```python
from build123d import *

# Parameters (mm, degrees)
SKETCH1_W                 = 47.35
SKETCH1_H                 = 43.25
BOSS_EXTRUDE2_DEPTH       = 2
EDGE_FLANGE1_START        = -2
EDGE_FLANGE1_OUTLINE_W    = 1
EDGE_FLANGE1_OUTLINE_H    = 2
EDGE_FLANGE1_DEPTH        = 2
EDGE_FLANGE1_START_2      = -1
EDGE_FLANGE1_2_DEPTH      = 3.69178
EDGE_FLANGE1_3_OUTLINE_W  = 2
EDGE_FLANGE1_3_OUTLINE_H  = 26.65
EDGE_FLANGE1_3_DEPTH      = 12
EDGE_FLANGE1_START_3      = 8.3
EDGE_FLANGE1_4_DEPTH      = 26.65
EDGE_FLANGE1_5_DEPTH      = 26.65
EDGE_FLANGE1_START_4      = 47.35
EDGE_FLANGE1_6_OUTLINE_R  = 1.6
EDGE_FLANGE1_6_DEPTH      = 2
REDONDEO1_R               = 2
TALADRO_ROSCADO_M31_D     = 2.5
TALADRO_ROSCADO_M31_DEPTH = 8.5
TALADRO_ROSCADO_M31_TIP   = 0.751075774
CROQUIS4_W                = 37.35
CROQUIS4_H                = 34.25
CORTAR_EXTRUIR1_DEPTH     = 67.377594111
CROQUIS14_W               = 2
CROQUIS14_H               = 7.3
SALIENTE_EXTRUIR1_DEPTH   = 1
FILLET1_R                 = 2
REDONDEO2_R               = 5
REDONDEO3_R               = 1


with BuildPart() as part:
    # Sketch1 → Boss-Extrude2 (new body)
    with BuildSketch(Plane.XY):
        with Locations((23.675, 21.625)):
            Rectangle(SKETCH1_W, SKETCH1_H)
    extrude(amount=BOSS_EXTRUDE2_DEPTH)

    # Edge-Flange1: read off the stored shape, not the designer's step
    # Edge-Flange1 outline → Edge-Flange1 (cut)
    with BuildSketch(Plane(origin=(47.35, 0, 2), x_dir=(0, 1, 0), z_dir=(1, 0, 0)).offset(EDGE_FLANGE1_START)):
        with Locations((35.45, -1)):
            Rectangle(EDGE_FLANGE1_OUTLINE_W, EDGE_FLANGE1_OUTLINE_H)
        with Locations((7.8, -1)):
            Rectangle(EDGE_FLANGE1_OUTLINE_W, EDGE_FLANGE1_OUTLINE_H)
    extrude(amount=EDGE_FLANGE1_DEPTH, mode=Mode.SUBTRACT)

    # Edge-Flange1 2 outline → Edge-Flange1 2 (cut)
    with BuildSketch(Plane.XY.offset(EDGE_FLANGE1_START_2)):
        with BuildLine():
            ThreePointArc((45.35, 35.95), (44.85, 35.45), (45.35, 34.95))
            Line((45.35, 34.95), (45.35, 35.95))
        make_face()
        with BuildLine():
            ThreePointArc((45.35, 8.3), (44.85, 7.8), (45.35, 7.3))
            Line((45.35, 7.3), (45.35, 8.3))
        make_face()
    extrude(amount=EDGE_FLANGE1_2_DEPTH, mode=Mode.SUBTRACT)

    # Edge-Flange1 3 outline → Edge-Flange1 3 (add)
    with BuildSketch(Plane.XY):
        with Locations((48.35, 21.625)):
            Rectangle(EDGE_FLANGE1_3_OUTLINE_W, EDGE_FLANGE1_3_OUTLINE_H)
    extrude(amount=EDGE_FLANGE1_3_DEPTH)

    # Edge-Flange1 4 outline → Edge-Flange1 4 (add)
    with BuildSketch(Plane(origin=(0, 0, 0), x_dir=(1, 0, 0), z_dir=(0, 1, 0)).offset(EDGE_FLANGE1_START_3)):
        with BuildLine():
            ThreePointArc((46.35, -2), (47.057106781, -2.292893219), (47.35, -3))
            Line((47.35, -3), (47.35, -2))
            Line((47.35, -2), (46.35, -2))
        make_face()
    extrude(amount=EDGE_FLANGE1_4_DEPTH)

    # Edge-Flange1 5 outline → Edge-Flange1 5 (cut)
    with BuildSketch(Plane(origin=(0, 0, 0), x_dir=(1, 0, 0), z_dir=(0, 1, 0)).offset(EDGE_FLANGE1_START_3)):
        with BuildLine():
            ThreePointArc((46.35, 0), (48.471320344, -0.878679656), (49.35, -3))
            Line((49.35, -3), (49.35, 0))
            Line((49.35, 0), (46.35, 0))
        make_face()
    extrude(amount=EDGE_FLANGE1_5_DEPTH, mode=Mode.SUBTRACT)

    # Edge-Flange1 6 outline → Edge-Flange1 6 (cut)
    with BuildSketch(Plane.YZ.offset(EDGE_FLANGE1_START_4)):
        with Locations((12.3, 8.5)):
            Circle(EDGE_FLANGE1_6_OUTLINE_R)
        with Locations((30.95, 8.5)):
            Circle(EDGE_FLANGE1_6_OUTLINE_R)
    extrude(amount=EDGE_FLANGE1_6_DEPTH, mode=Mode.SUBTRACT)

    # Redondeo1
    redondeo1_edges = [part.edges().sort_by_distance(p)[0] for p in [
        (48.35, 8.3, 12),
        (48.35, 34.95, 12),
    ]]
    fillet(redondeo1_edges, radius=REDONDEO1_R)

    # Taladro roscado M31
    with Locations(Plane(origin=(0, 0, 0), x_dir=(-1, 0, 0), z_dir=(0, 0, -1))):
        with Locations((-44.65, 39.45), (-4, 3.8), (-44.65, 3.8)):
            Hole(TALADRO_ROSCADO_M31_D / 2, depth=TALADRO_ROSCADO_M31_DEPTH)
            with Locations((0, 0, -(TALADRO_ROSCADO_M31_DEPTH + TALADRO_ROSCADO_M31_TIP / 2))):  # 118° drill point
                Cone(0, TALADRO_ROSCADO_M31_D / 2, TALADRO_ROSCADO_M31_TIP, mode=Mode.SUBTRACT)

    # Croquis4 → Cortar-Extruir1 (cut, through all)
    with BuildSketch(Plane.XY.offset(2)):
        with Locations((18.675, 26.125)):
            Rectangle(CROQUIS4_W, CROQUIS4_H)
    extrude(amount=-CORTAR_EXTRUIR1_DEPTH, mode=Mode.SUBTRACT)

    # Croquis14 → Saliente-Extruir1 (add)
    with BuildSketch(Plane(origin=(47.35, 0, 0), x_dir=(0, 0, -1), z_dir=(1, 0, 0))):
        with Locations((-1, 3.65)):
            Rectangle(CROQUIS14_W, CROQUIS14_H)
        with Locations((-1, 39.6)):
            Rectangle(CROQUIS14_W, CROQUIS14_H)
    extrude(amount=SALIENTE_EXTRUIR1_DEPTH)

    # Fillet1
    fillet1_edges = [part.edges().sort_by_distance(p)[0] for p in [
        (0, 9, 1),
        (37.35, 43.25, 1),
        (48.35, 0, 1),
        (48.35, 43.25, 1),
        (0, 0, 1),
    ]]
    fillet(fillet1_edges, radius=FILLET1_R)

    # Redondeo2
    redondeo2_edges = [part.edges().sort_by_distance(p)[0] for p in [
        (37.35, 9, 1),
    ]]
    fillet(redondeo2_edges, radius=REDONDEO2_R)

    # Redondeo3
    redondeo3_edges = [part.edges().sort_by_distance(p)[0] for p in [
        (48.35, 7.3, 1),
        (48.35, 35.95, 1),
    ]]
    fillet(redondeo3_edges, radius=REDONDEO3_R)


solid = part.part
```
The model under review builds one solid part; all positions refer to its coordinate system, in mm. A direction names the side the tool comes from. Give positions to 0.01 mm unless a question says otherwise; leave off trailing zeros. Write each loop counter-clockwise with the first axis right and the second up, starting at its lowest first coordinate (ties: lowest second). Pieces come first, ordered by that corner, then holes. Notation, with made-up numbers: (78.5, 77.5) - (114.5, 77.5) arc R20 ccw to (114.5, 90.5) - close; hole circle Ø11 at (6.5, 86.25). An arc over 180 degrees is marked (long way). Answer in a Markdown table with one row per item. Add a question column.
1. We need section B-B on y = 39.45. Write out the cut boundary in (x, z), then the cut area to 3 significant figures.
2. We need section A-A on x = 4. Write out the cut boundary in (y, z), then the cut area to 3 significant figures.
3. We need section D-D on z = 4. Write out the cut boundary in (x, y).
4. Draft analysis for pull direction X (two halves, no side actions). For faces 5 (the flat face through (29, 7, 0)), 6 (the flat face through (48.35, 4, 1)), 7 (the cylindrical face through (5.19, 4.18, 1.01)), state which applies: +X half, -X half, draft (parallel to the pull), parting line (faces both ways), or undercut.
5. We need section C-C on y = 25.5. Write out the cut boundary in (x, z), then the cut area to 3 significant figures.
6. Wall thickness on line 1 along Y through (x, z) = (44.65, 0.65); line 2 along Z through (x, y) = (16, 7); line 3 along Z through (x, y) = (48.7, 12.3): over which ranges is each line inside the solid? List them lowest first. Write a range as [from, to].
7. Tool access review of faces 1 (the flat face through (46, 35.95, 1)), 2 (the flat face through (37.35, 27, 1)), 3 (the cylindrical face through (48.45, 21.44, 0.86)), 4 (the cylindrical face through (47.75, 0.57, 0.99)): name each direction out of +Z, -Z, +X, -X, +Y, -Y from which nothing blocks a thin tool from reaching the whole face with its end or side.
8. Insertion check: P1, Ø2, axis at x = 47.5, z = 6.5, coming from the +Y side; P2, Ø2, axis at y = 4.5, z = 1, coming from the +X side; P3, Ø6, axis at y = 32.5, z = 10, coming from the -X side; P4, Ø3, axis at y = 37.5, z = 10.5, coming from the +X side. Each pin has a flat end and moves straight along its axis. Give the tip position at first contact, or say it passes through.
Ans:
| question | item | result |
|---|---|---|
| 1 | outline | (37.35, 0) - (43.4, 0) - (43.4, 2) - (37.35, 2) - close; (45.9, 0) - (48.35, 0) - (48.35, 2) - (45.9, 2) - close |
| 1 | area | 17.0 mm^2 |
| 2 | outline | (0, 0) - (2.55, 0) - (2.55, 2) - (0, 2) - close; (5.05, 0) - (9, 0) - (9, 2) - (5.05, 2) - close |
| 2 | area | 13.0 mm^2 |
| 3 | outline | (47.35, 8.3) - (49.35, 8.3) - (49.35, 34.95) - (47.35, 34.95) - close |
| 4 | face 5 | draft |
| 4 | face 6 | +X half |
| 4 | face 7 | undercut |
| 5 | outline | (37.35, 0) - (46.35, 0) arc R3 ccw to (49.35, 3) - (49.35, 12) - (47.35, 12) - (47.35, 3) arc R1 cw to (46.35, 2) - (37.35, 2) - close |
| 5 | area | 42.3 mm^2 |
| 6 | line 1 | y = [0, 2.55], [5.05, 38.2], [40.7, 43.25] |
| 6 | line 2 | z = [0, 2] |
| 6 | line 3 | z = [1.14, 6.9], [10.1, 12] |
| 7 | face 1 | +Z, -Z, +X |
| 7 | face 2 | +Z, -Z, -X, +Y |
| 7 | face 3 | -Z, +X |
| 7 | face 4 | +Z, -Z, +X, -Y |
| 8 | P1 | stops at y = 34.95 |
| 8 | P2 | stops at x = 48.35 |
| 8 | P3 | stops at x = 47.35 |
| 8 | P4 | passes through |
